from build123d import *

# Parameters (mm, degrees)
SKETCH1_R           = 38.1
BOSS_EXTRUDE1_DEPTH = 2.54
SKETCH3_R           = 6.35
BOSS_EXTRUDE3_DEPTH = 19.05
SKETCH2_R           = 3.429
CUT_EXTRUDE1_DEPTH  = 59.046086001
CUT_EXTRUDE2_DEPTH  = 59.046086001


with BuildPart() as part:
    # Sketch1 → Boss-Extrude1 (new body)
    with BuildSketch(Plane.XY):
        Circle(SKETCH1_R)
    extrude(amount=BOSS_EXTRUDE1_DEPTH)

    # Sketch3 → Boss-Extrude3 (add)
    with BuildSketch(Plane(origin=(0, 0, 0), x_dir=(-1, 0, 0), z_dir=(0, 0, -1))):
        with Locations(Location((0, 0, 0), (0, 0, 180))):
            Circle(SKETCH3_R)
    extrude(amount=BOSS_EXTRUDE3_DEPTH)

    # Sketch2 → Cut-Extrude1 (cut, through all)
    with BuildSketch(Plane.XY.offset(2.54)):
        with Locations((0, 30.48)):
            Circle(SKETCH2_R)
    extrude(amount=-CUT_EXTRUDE1_DEPTH, mode=Mode.SUBTRACT)

    # Sketch4 → Cut-Extrude2 (cut, through all)
    with BuildSketch(Plane(origin=(0, 0, -19.05), x_dir=(-1, 0, 0), z_dir=(0, 0, -1))):
        with BuildLine():
            Line((-2.076655966, 2.5), (2.076655966, 2.5))
            ThreePointArc((2.076655966, 2.5), (0, -3.25), (-2.076655966, 2.5))
        make_face()
    extrude(amount=-CUT_EXTRUDE2_DEPTH, mode=Mode.SUBTRACT)


solid = part.part
Here's how the part is built. I have some questions about the finished solid (model axes, mm). A direction names the side the tool comes from. Coordinates: 2 decimals unless noted, no trailing zeros. Order: outer loops, then holes, each group sorted by start corner. A loop starts at its lowest first (then second) coordinate and runs counter-clockwise, first axis right, second up. Notation, with made-up numbers: (50.5, 34.5) - (102.5, 34.5) arc R8 ccw to (102.5, 49.5) - close; hole circle Ø3 at (-19, 54). An arc over 180 degrees is marked (long way). Use CSV: the item, a comma, the result in double quotes. Start each with the question number.
1. For faces 4 (the face through (2.93, 5.634, -9.392)), 5 (the face through (0, 2.5, -8)), 6 (the face through (8, 1, 2.54)), which set-ups out of +Z, -Z, +X, -X, +Y, -Y let a thin tool reach every point of the face, with its end or its side?
2. I'm going to push flat-ended pins straight in: pin 1 (5 mm diameter, centred on x = 2, z = -1.5, fed in from +Y); pin 2 (1.5 mm diameter, centred on x = -16, y = 7, fed in from -Z); pin 3 (10 mm diameter, centred on x = 1.5, z = -15, fed in from -Y). Where does each tip first touch, or does it pass through?
3. Please list where these lines run through material, in increasing order: line 1 (Y direction, x = 0, z = 1.3); line 2 (Y direction, x = 0, z = -14.5); line 3 (Z direction, x = -17, y = -14). Write a range as from..to.
4. Suppose I cut it at C-C on z = 1.25. List the corners of the cut face in (x, y) for me, then the cut area to 3 significant figures.
5. Suppose I cut it at D-D on z = -6.5. List the corners of the cut face in (x, y) for me, then the cut area to 3 significant figures.
6. Suppose I cut it at A-A on x = 0. List the corners of the cut face in (y, z) for me.
7. Suppose I cut it at B-B on y = 30.48. List the corners of the cut face in (x, z) for me.
8. If we mould it in two halves opening along Y, with no side actions, what happens to faces 1 (the face through (1.8, 33.4, 1.3)), 2 (the face through (0, 3, -19.05)), 3 (the face through (-30.235, -23.183, 1.252))? For each: +Y half, -Y half, draft (parallel to the pull), parting line (faces both ways), or undercut.
Output:
1,face 4,"-Z"
1,face 5,"+Z, -Z"
1,face 6,"+Z, +X, -X, +Y, -Y"
2,pin 1,"stops at y = 38.1"
2,pin 2,"stops at z = 0"
2,pin 3,"stops at y = -6.35"
3,line 1,"y = -38.1..-3.25, 2.5..27.05, 33.91..38.1"
3,line 2,"y = -6.35..-3.25, 2.5..6.35"
3,line 3,"z = 0..2.54"
4,outline,"circle Ø76.2 at (0, 0); hole circle Ø6.86 at (0, 30.48); hole (-2.08, 2.5) arc R3.25 ccw (long way) to (2.08, 2.5) - close"
4,area,"4,490 mm2"
5,outline,"circle Ø12.7 at (0, 0); hole (-2.08, 2.5) arc R3.25 ccw (long way) to (2.08, 2.5) - close"
5,area,"95.6 mm2"
6,outline,"(-38.1, 0) - (-6.35, 0) - (-6.35, -19.05) - (-3.25, -19.05) - (-3.25, 2.54) - (-38.1, 2.54) - close; (2.5, -19.05) - (6.35, -19.05) - (6.35, 0) - (27.05, 0) - (27.05, 2.54) - (2.5, 2.54) - close; (33.91, 0) - (38.1, 0) - (38.1, 2.54) - (33.91, 2.54) - close"
7,outline,"(-22.86, 0) - (-3.43, 0) - (-3.43, 2.54) - (-22.86, 2.54) - close; (3.43, 0) - (22.86, 0) - (22.86, 2.54) - (3.43, 2.54) - close"
8,face 1,"undercut"
8,face 2,"draft"
8,face 3,"parting line"
